from build123d import *

# Parameters (mm, degrees)
SKIZZE1_R                       = 2.5
AUFSATZ_LINEAR_AUSTRAGEN1_DEPTH = 6
SKIZZE2_R                       = 4.5
SCHNITT_LINEAR_AUSTRAGEN1_DEPTH = 4
SKIZZE3_R                       = 8
SCHNITT_LINEAR_AUSTRAGEN2_DEPTH = 4


with BuildPart() as part:
    # Skizze1 → Aufsatz-Linear austragen1 (new body)
    with BuildSketch(Plane.XY):
        Polygon((16, 9.237604307), (0, 18.475208614), (-16, 9.237604307), (-16, -9.237604307), (0, -18.475208614), (16, -9.237604307), align=None)
        Circle(SKIZZE1_R, mode=Mode.SUBTRACT)
    extrude(amount=AUFSATZ_LINEAR_AUSTRAGEN1_DEPTH)

    # Skizze2 → Schnitt-Linear austragen1 (cut)
    with BuildSketch(Plane.XY.offset(6)):
        Circle(SKIZZE2_R)
    extrude(amount=-SCHNITT_LINEAR_AUSTRAGEN1_DEPTH, mode=Mode.SUBTRACT)

    # Skizze3 → Schnitt-Linear austragen2 (cut)
    with BuildSketch(Plane(origin=(0, 0, 0), x_dir=(-1, 0, 0), z_dir=(0, 0, -1))):
        Polygon((13.971876514, 0), (6.985938257, 12.1), (-6.985938257, 12.1), (-13.971876514, 0), (-6.985938257, -12.1), (6.985938257, -12.1), align=None)
        Circle(SKIZZE3_R, mode=Mode.SUBTRACT)
    extrude(amount=-SCHNITT_LINEAR_AUSTRAGEN2_DEPTH, mode=Mode.SUBTRACT)


solid = part.part
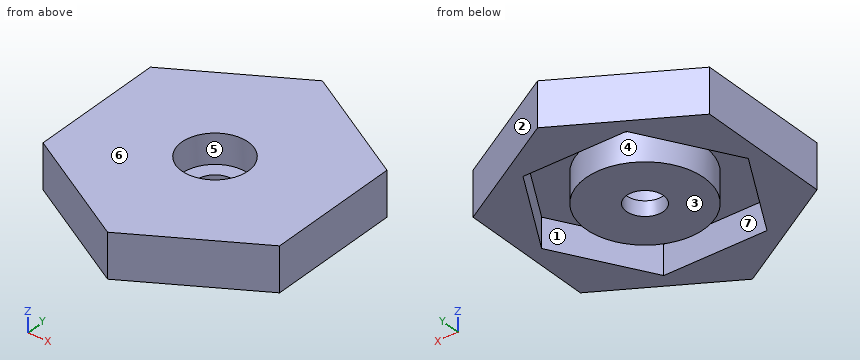
For this review, take the finished solid that the model builds, in its own axes (mm). Face numbers are marked on the shaded views. A direction names the side the tool comes from. Give positions to 0.01 mm unless a question says otherwise; leave off trailing zeros. Loops run counter-clockwise (first coordinate to the right, second up) from the corner with the lowest first, then second, coordinate; pieces in that order, holes last.
Item 1: For line 1 along Y through (x, z) = (0, 2.75); line 2 along Y through (x, z) = (0, 1); line 3 along Z through (x, y) = (4.5, 7.5), list the stretches that pass through material, from the lowest coordinate up.
Item 2: Take a section at D-D, the plane x = -13. State the section outline as (y, z) points.
Item 3: Insertion check: pin 1 (3 mm diameter, centred on x = 5, z = 3, fed in from -Y); pin 2 (1.5 mm diameter, centred on x = 8, y = 5, fed in from -Z); pin 3 (1.2 mm diameter, centred on x = 3.5, z = 2.5, fed in from +Y). Each pin has a flat end and moves straight along its axis. Give the tip position at first contact, or say it passes through.
Item 4: Take a section at B-B, the plane x = 1. State the section outline as (y, z) points, and give its area (3 significant figures).
Item 5: Draft analysis for pull direction Y (two halves, no side actions). For the marked faces 1, 2, 3 and 4, state which applies: +Y half, -Y half, draft (parallel to the pull), parting line (faces both ways), or undercut.
Item 6: Take a section at A-A, the plane z = 2.7. State the section outline as (x, y) points, and give its area (3 significant figures).
Item 7: Take a section at C-C, the plane y = 3.5. State the section outline as (x, z) points.
Item 8: Tool access review of the marked faces 5, 6 and 7: name each direction out of +Z, -Z, +X, -X, +Y, -Y from which nothing blocks a thin tool from reaching the whole face with its end or side.
Calculated:
1. line 1: y = -18.48 to -12.1, -8 to -4.5, 4.5 to 8, 12.1 to 18.48
1. line 2: y = -18.48 to -12.1, -8 to -2.5, 2.5 to 8, 12.1 to 18.48
1. line 3: z = 4 to 6
2. outline: (-10.97, 0) - (-1.68, 0) - (-1.68, 4) - (1.68, 4) - (1.68, 0) - (10.97, 0) - (10.97, 6) - (-10.97, 6) - close
3. pin 1: stops at y = -16.45
3. pin 2: stops at z = 4
3. pin 3: stops at y = 16.8
4. outline: (-17.9, 0) - (-12.1, 0) - (-12.1, 4) - (-7.94, 4) - (-7.94, 0) - (-2.29, 0) - (-2.29, 2) - (-4.39, 2) - (-4.39, 6) - (-17.9, 6) - close; (2.29, 0) - (7.94, 0) - (7.94, 4) - (12.1, 4) - (12.1, 0) - (17.9, 0) - (17.9, 6) - (4.39, 6) - (4.39, 2) - (2.29, 2) - close
4. area: 137 mm2
5. face 1: undercut
5. face 2: +Y half
5. face 3: draft
5. face 4: undercut
6. outline: (-16, -9.24) - (0, -18.48) - (16, -9.24) - (16, 9.24) - (0, 18.48) - (-16, 9.24) - close; circle Ø16 at (0, 0); hole (-13.97, 0) - (-6.99, -12.1) - (6.99, -12.1) - (13.97, 0) - (6.99, 12.1) - (-6.99, 12.1) - close; hole circle Ø9 at (0, 0)
6. area: 517 mm2
7. outline: (-16, 0) - (-11.95, 0) - (-11.95, 4) - (-7.19, 4) - (-7.19, 0) - (7.19, 0) - (7.19, 4) - (11.95, 4) - (11.95, 0) - (16, 0) - (16, 6) - (2.83, 6) - (2.83, 2) - (-2.83, 2) - (-2.83, 6) - (-16, 6) - close
8. face 5: +Z
8. face 6: +Z, +X, -X, +Y, -Y
8. face 7: -Z
